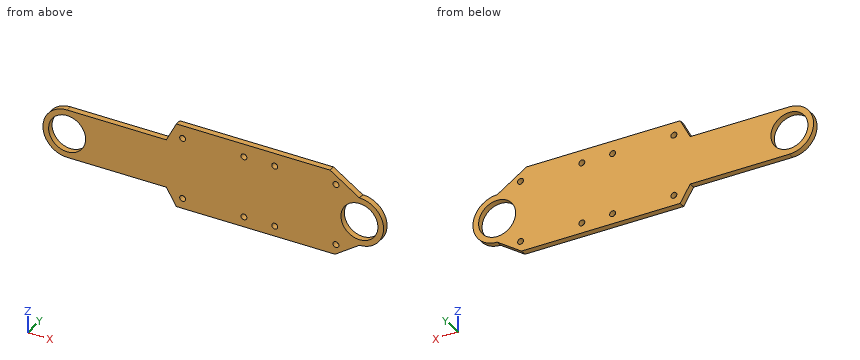
```python
from build123d import *

# Parameters (mm, degrees)
SKETCH5_W          = 50.68
SKETCH5_H          = 3.06
EXTRUDE2_DEPTH     = 180
SKETCH6_R          = 9.36
SKETCH6_R_2        = 1.5
CUT_EXTRUDE3_DEPTH = 182.800657865
SKETCH7_W          = 77.752773683
SKETCH7_H          = 3.335005788
CUT_EXTRUDE4_DEPTH = 178.825100476


with BuildPart() as part:
    # Sketch5 → Extrude2 (new body)
    with BuildSketch(Plane(origin=(0, 0, 0), x_dir=(0, 0, -1), z_dir=(1, 0, 0))):
        Rectangle(SKETCH5_W, SKETCH5_H)
    extrude(amount=EXTRUDE2_DEPTH)

    # Sketch6 → Cut-Extrude3 (cut, through all)
    with BuildSketch(Plane(origin=(0, 1.53, 0), x_dir=(-1, 0, 0), z_dir=(0, 1, 0))):
        with Locations(Location((-15.875, 0, 0), (0, 0, 90))):
            Circle(SKETCH6_R)
        with Locations(Location((-74.32, -15.5, 0), (0, 0, 90))):
            Circle(SKETCH6_R_2)
        with Locations(Location((-74.32, 15.5, 0), (0, 0, 90))):
            Circle(SKETCH6_R_2)
        with Locations(Location((-105.32, -15.5, 0), (0, 0, 90))):
            Circle(SKETCH6_R_2)
        with Locations(Location((-105.32, 15.5, 0), (0, 0, 90))):
            Circle(SKETCH6_R_2)
        with Locations(Location((-120.9, -15.5, 0), (0, 0, 90))):
            Circle(SKETCH6_R_2)
        with Locations(Location((-120.9, 15.5, 0), (0, 0, 90))):
            Circle(SKETCH6_R_2)
        with Locations(Location((-151.9, -15.5, 0), (0, 0, 90))):
            Circle(SKETCH6_R_2)
        with Locations(Location((-151.9, 15.5, 0), (0, 0, 90))):
            Circle(SKETCH6_R_2)
        with Locations(Location((-163.76, 0, 0), (0, 0, 90))):
            Circle(SKETCH6_R)
        with BuildLine():
            Line((-163.76, 12.223769591), (-148.9, 22.004994212))
            Line((-148.9, 22.004994212), (-148.9, 25.34))
            Line((-148.9, 25.34), (-180, 25.34))
            Line((-180, 25.34), (-180, -25.34))
            Line((-180, -25.34), (0, -25.34))
            Line((0, -25.34), (0, 25.34))
            Line((0, 25.34), (-71.147226317, 25.34))
            Line((-71.147226317, 25.34), (-71.147226317, 22.004994212))
            Line((-71.147226317, 22.004994212), (-66.075480217, 12.223769591))
            Line((-66.075480217, 12.223769591), (-15.875, 12.223769591))
            ThreePointArc((-15.875, 12.223769591), (-3.651230409, 0), (-15.875, -12.223769591))
            Line((-15.875, -12.223769591), (-66.075480217, -12.223769591))
            Line((-66.075480217, -12.223769591), (-71.147226317, -20.64))
            Line((-71.147226317, -20.64), (-151.43711062, -20.64))
            Line((-151.43711062, -20.64), (-163.76, -12.223769591))
            ThreePointArc((-163.76, -12.223769591), (-175.983769591, 0), (-163.76, 12.223769591))
        make_face()
    extrude(amount=-CUT_EXTRUDE3_DEPTH, mode=Mode.SUBTRACT)

    # Sketch7 → Cut-Extrude4 (cut, through all)
    with BuildSketch(Plane(origin=(0, 1.53, 0), x_dir=(-1, 0, 0), z_dir=(0, 1, 0))):
        with Locations((-110.023613159, 23.672497106)):
            Rectangle(SKETCH7_W, SKETCH7_H)
    extrude(amount=-CUT_EXTRUDE4_DEPTH, mode=Mode.SUBTRACT)


solid = part.part
```
The listing builds one solid part. Answer for the finished solid, in the listing's coordinates (mm). Coordinates: 2 decimals unless noted, no trailing zeros. Loops run counter-clockwise (first coordinate to the right, second up) from the corner with the lowest first, then second, coordinate; pieces in that order, holes last. Notation, with made-up numbers: (16.5, 62) -> (61.5, 62) arc R9 cw to (61.5, 71) -> close; hole circle Ø10 at (6, -14.75). An arc over 180 degrees is marked (long way). Return JSON: item names as keys, results as strings. Group by question number.
(1) A cutting plane is placed at A-A on x = 74.32. Write down the section's boundary in (y, z) (3 decimals), and give its area (3 significant figures).
(2) A cutting plane is placed at B-B on z = 0. Write down the section's boundary in (x, y) (3 decimals), and give its area (3 significant figures).
(3) Given pin 1 Ø5 at (x, z) = (120.9, -15.5) entering from -Y; pin 2 Ø0.9 at (x, y) = (46, 0) entering from -Z, each flat-ended and moving along its own axis, determine where each tip first touches the part or whether it passes through.
(4) Find the intervals of material crossed by probe 1 along Z at (x, y) = (105.32, 0.3) (3 decimals); probe 2 along X at (y, z) = (-0.75, -1); probe 3 along X at (y, z) = (-0.4, -2.5), in increasing order. Write a range as from..to.
(5) A cutting plane is placed at D-D on z = -15.5. Write down the section's boundary in (x, y), and give its area (3 significant figures).
(6) A cutting plane is placed at C-C on y = 0.7. Count the separate pieces of the cut face and the enclosed holes in it, and give its area (3 significant figures).
The answers:
{
 "1": {"outline": "(-1.53, -20.64) -> (1.53, -20.64) -> (1.53, -17) -> (-1.53, -17) -> close; (-1.53, -14) -> (1.53, -14) -> (1.53, 14) -> (-1.53, 14) -> close; (-1.53, 17) -> (1.53, 17) -> (1.53, 22.005) -> (-1.53, 22.005) -> close", "area": "112 mm^2"},
 "2": {"outline": "(3.651, -1.53) -> (6.515, -1.53) -> (6.515, 1.53) -> (3.651, 1.53) -> close; (25.235, -1.53) -> (154.4, -1.53) -> (154.4, 1.53) -> (25.235, 1.53) -> close; (173.12, -1.53) -> (175.984, -1.53) -> (175.984, 1.53) -> (173.12, 1.53) -> close", "area": "413 mm^2"},
 "3": {"pin 1": "stops at y = -1.53", "pin 2": "stops at z = -12.22"},
 "4": {"probe 1": "z = -20.64..-17, -14..14, 17..22.005", "probe 2": "x = 3.69..6.57, 25.18..154.45, 173.07..175.94", "probe 3": "x = 3.91..6.86, 24.89..154.74, 172.78..175.73"},
 "5": {"outline": "(68.05, -1.53) -> (72.82, -1.53) -> (72.82, 1.53) -> (68.05, 1.53) -> close; (75.82, -1.53) -> (103.82, -1.53) -> (103.82, 1.53) -> (75.82, 1.53) -> close; (106.82, -1.53) -> (119.4, -1.53) -> (119.4, 1.53) -> (106.82, 1.53) -> close; (122.4, -1.53) -> (150.4, -1.53) -> (150.4, 1.53) -> (122.4, 1.53) -> close; (153.4, -1.53) -> (158.96, -1.53) -> (158.96, 1.53) -> (153.4, 1.53) -> close", "area": "241 mm^2"},
 "6": {"separate pieces": "1", "enclosed holes": "10", "area": "5,080 mm^2"}
}
